```python
from build123d import *

# Parameters (mm, degrees)
F0_W     = 30
F0_H     = 11
F1_DEPTH = 3
F2_SIZE2 = 2.99999
F2_SIZE  = 2.99999
F3_D     = 3.3


# Not quite as in the source:
# - a fillet or chamfer is up to 0.001 mm smaller than in the source, because OpenCascade refuses the exact size


with BuildPart() as f1:
    # F0 (on Top) → F1 (new body)
    with BuildSketch(Plane.XY):
        with Locations((15, -5.5)):
            Rectangle(F0_W, F0_H)
    extrude(amount=F1_DEPTH)

    # F2 (size 3 and 3 in the source; OpenCascade refuses exactly that, so slightly less here)
    f2_edges = [f1.edges().sort_by_distance(p)[0] for p in [
        (15, -11, 3),
        (15, 0, 3),
    ]]
    chamfer(f2_edges, length=F2_SIZE, length2=F2_SIZE2)

    # F3 (through all)
    with Locations(Plane(origin=(0, 0, 0), x_dir=(1, 0, 0), z_dir=(0, 0, -1))):
        with Locations((4, 5.5), (26, 5.5)):
            Hole(F3_D / 2)


solid = f1.part
```
For this review, take the finished solid that the model builds, in its own axes (mm). Round coordinates to 2 decimals unless told otherwise and drop trailing zeros. Write each loop counter-clockwise with the first axis right and the second up, starting at its lowest first coordinate (ties: lowest second). Pieces come first, ordered by that corner, then holes. Notation, with made-up numbers: (85, 78.5) -> (116, 78.5) arc R28 ccw to (116, 109.5) -> close; hole circle Ø2 at (-15.5, 28.25). An arc over 180 degrees is marked (long way). Use one line per item in the form item = value.
1) Clearance check with a flat-ended pin moving along its axis: pin 1 (1 mm diameter, centred on x = 3, z = 2, fed in from -Y). State where the tip first meets the part, or that it passes through.
Found:
pin_1 = -9.5
2) Mouldability with a two-part tool opening along Y and no side actions: class faces 1 (the flat face through (15, -2, 2)), 2 (the cylindrical face through (5.31, -4.5, 1.52)), 3 (the flat face through (15, -5, 0)) as +Y half, -Y half, draft (parallel to the pull), parting line (faces both ways), or undercut.
Found:
face_1 = +Y half
face_2 = undercut
face_3 = draft
3) To check wall thickness, follow L1, parallel to X at y = -5.5, z = 1.65; L2, parallel to Y at x = 4.75, z = 1.5; L3, parallel to X at y = -4.75, z = 2.15. State the ranges of each line that lie inside material, in increasing order. Write a range as from..to.
Found:
L1 = 0..2.35, 5.65..24.35, 27.65..30
L2 = -9.5..-6.97, -4.03..-1.5
L3 = 0..2.53, 5.47..24.53, 27.47..30
4) Take a section at C-C, the plane y = -4.75. Write out the cut boundary in (x, z).
Found:
outline = (0, 0) -> (2.53, 0) -> (2.53, 3) -> (0, 3) -> close; (5.47, 0) -> (24.53, 0) -> (24.53, 3) -> (5.47, 3) -> close; (27.47, 0) -> (30, 0) -> (30, 3) -> (27.47, 3) -> close
5) Take a section at B-B, the plane z = 0.5. Write out the cut boundary in (x, y), and give its area (3 significant figures).
Found:
outline = (0, -10.5) -> (30, -10.5) -> (30, -0.5) -> (0, -0.5) -> close; hole circle Ø3.3 at (4, -5.5); hole circle Ø3.3 at (26, -5.5)
area = 283 mm2
